from build123d import *

# Parameters (mm, degrees)
AUFSATZ_LINEAR_AUSTRAGEN1_DEPTH                      = 5
VERRUNDUNG1_R                                        = 30
STIRNSENKUNG_F_R_M5_ZYLINDERSCHRAUBE_MIT_D           = 5.3
STIRNSENKUNG_F_R_M5_ZYLINDERSCHRAUBE_MIT_CBORE_D     = 10
STIRNSENKUNG_F_R_M5_ZYLINDERSCHRAUBE_MIT_CBORE_DEPTH = 5.4
LINEARES_MUSTER1_COUNT                               = 3
LINEARES_MUSTER1_PITCH                               = 30
LINEARES_MUSTER1_COUNT_DIR2                          = 2
LINEARES_MUSTER1_PITCH_DIR2                          = 50


with BuildPart() as part:
    # Skizze1 → Aufsatz-Linear austragen1 (new body, symmetric)
    with BuildSketch(Plane.XY):
        with BuildLine():
            Line((-120, 60), (0, 60))
            Line((0, 60), (0, -60))
            Line((0, -60), (-120, -60))
            ThreePointArc((-120, -60), (-100, 0), (-120, 60))
        make_face()
    extrude(amount=AUFSATZ_LINEAR_AUSTRAGEN1_DEPTH, both=True)

    # Verrundung1
    verrundung1_edges = [part.edges().sort_by_distance(p)[0] for p in [
        (0, 60, 0),
    ]]
    fillet(verrundung1_edges, radius=VERRUNDUNG1_R)

    # Stirnsenkung für M5 Zylinderschraube mit Innensechskant1 (through all)
    with Locations(Plane.XY.offset(5)):
        with Locations((-30, 30)):
            stirnsenkung_f_r_m5_zylinderschraube_mit = CounterBoreHole(STIRNSENKUNG_F_R_M5_ZYLINDERSCHRAUBE_MIT_D / 2, STIRNSENKUNG_F_R_M5_ZYLINDERSCHRAUBE_MIT_CBORE_D / 2, STIRNSENKUNG_F_R_M5_ZYLINDERSCHRAUBE_MIT_CBORE_DEPTH)

    # Lineares Muster1: Stirnsenkung f_r M5 Zylinderschraube mit 3 × 2
    with Locations(*[(-j * LINEARES_MUSTER1_PITCH_DIR2, -i * LINEARES_MUSTER1_PITCH, 0) for i in range(LINEARES_MUSTER1_COUNT) for j in range(LINEARES_MUSTER1_COUNT_DIR2) if (i, j) != (0, 0)]):
        add(stirnsenkung_f_r_m5_zylinderschraube_mit, mode=Mode.SUBTRACT)


solid = part.part
Design review of the part built by this model. Coordinates are the model's own, in mm. A direction names the side the tool comes from. Give positions to 0.01 mm unless a question says otherwise; leave off trailing zeros. Write each loop counter-clockwise with the first axis right and the second up, starting at its lowest first coordinate (ties: lowest second). Pieces come first, ordered by that corner, then holes. Notation, with made-up numbers: M 13,45.25 L 23,45.25 A14 ccw 23,64.25 Z; hole C 33.25,12.5 d1. An arc over 180 degrees is marked long. Answer as a JSON object with one key per item and string values. Group by question number.
1) Clearance check with flat-ended pins moving along their axes: pin 1 Ø1 at (y, z) = (23.5, -2) entering from -X; pin 2 Ø1 at (y, z) = (-35.5, 3) entering from -X; pin 3 Ø6 at (x, y) = (-80, 0) entering from +Z; pin 4 Ø3 at (x, y) = (-80.5, -30) entering from +Z. State where each tip first meets the part, or that it passes through.
2) We need section C-C (x = -80). Give the boundary of the cut face in (y, z).
3) Tool access review of faces 1 (the face through (-28, -32, -0.4)), 2 (the face through (-28.047, 31.791, -2.732)): name each direction out of +Z, -Z, +X, -X, +Y, -Y from which nothing blocks a thin tool from reaching the whole face with its end or side.
4) For line 1 along Y through (x, z) = (-80, 2.7); line 2 along Y through (x, z) = (-29, 2.75); line 3 along X through (y, z) = (31.5, 1.75), list the stretches that pass through material, from the lowest coordinate up.
5) We need section B-B (z = 3.5). Give the boundary of the cut face in (x, y), and give its area (3 significant figures).
6) We need section A-A (y = 0). Give the boundary of the cut face in (x, z), and give its area (3 significant figures).
7) We need section D-D (y = -30). Give the boundary of the cut face in (x, z).
8) Mouldability with a two-part tool opening along Y and no side actions: class faces 3 (the face through (-59, 1, 5)), 4 (the face through (-76, 60, 0)), 5 (the face through (-82.528, 0.796, -2.732)) as released by +Y, released by -Y, zero draft, split by the parting line, or undercut.
Answer key:
{
 "1": {"pin 1": "stops at x = -102.92", "pin 2": "stops at x = -106.7", "pin 3": "stops at z = -0.4", "pin 4": "passes through"},
 "2": {"outline": "M -60,-5 L -32.65,-5 L -32.65,-0.4 L -35,-0.4 L -35,5 L -60,5 Z; M -27.35,-5 L -2.65,-5 L -2.65,-0.4 L -5,-0.4 L -5,5 L -25,5 L -25,-0.4 L -27.35,-0.4 Z; M 2.65,-5 L 27.35,-5 L 27.35,-0.4 L 25,-0.4 L 25,5 L 5,5 L 5,-0.4 L 2.65,-0.4 Z; M 32.65,-5 L 60,-5 L 60,5 L 35,5 L 35,-0.4 L 32.65,-0.4 Z"},
 "3": {"face 1": "+Z", "face 2": "+Z, -Z"},
 "4": {"line 1": "y = -60 to -35, -25 to -5, 5 to 25, 35 to 60", "line 2": "y = -60 to -34.9, -25.1 to -4.9, 4.9 to 25.1, 34.9 to 59.98", "line 3": "x = -105.09 to -84.77, -75.23 to -34.77, -25.23 to -0.04"},
 "5": {"outline": "M -120,-60 L 0,-60 L 0,30 A30 ccw -30,60 L -120,60 A100 cw Z; hole C -80,-30 d10; hole C -80,0 d10; hole C -80,30 d10; hole C -30,-30 d10; hole C -30,0 d10; hole C -30,30 d10", "area": "12,100 mm²"},
 "6": {"outline": "M -100,-5 L -82.65,-5 L -82.65,-0.4 L -85,-0.4 L -85,5 L -100,5 Z; M -77.35,-5 L -32.65,-5 L -32.65,-0.4 L -35,-0.4 L -35,5 L -75,5 L -75,-0.4 L -77.35,-0.4 Z; M -27.35,-5 L 0,-5 L 0,5 L -25,5 L -25,-0.4 L -27.35,-0.4 Z", "area": "843 mm²"},
 "7": {"outline": "M -104.61,-5 L -82.65,-5 L -82.65,-0.4 L -85,-0.4 L -85,5 L -104.61,5 Z; M -77.35,-5 L -32.65,-5 L -32.65,-0.4 L -35,-0.4 L -35,5 L -75,5 L -75,-0.4 L -77.35,-0.4 Z; M -27.35,-5 L 0,-5 L 0,5 L -25,5 L -25,-0.4 L -27.35,-0.4 Z"},
 "8": {"face 3": "zero draft", "face 4": "released by +Y", "face 5": "undercut"}
}
